Source: CAD feature listing. Evaluate the final solid. Frame: model axes, mm. Face numbers are marked on the shaded views. A direction names the side the tool comes from. Give positions to 0.01 mm unless a question says otherwise; leave off trailing zeros. Write each loop counter-clockwise with the first axis right and the second up, starting at its lowest first coordinate (ties: lowest second). Pieces come first, ordered by that corner, then holes. Notation, with made-up numbers: (48, -26.5) -> (66, -26.5) arc R21 ccw to (66, 11.5) -> close; hole circle Ø1 at (30, -1.75). An arc over 180 degrees is marked (long way). Write item = value, one per line.
Autodesk Inventor part; units mm, degrees
ref_plane "YZ Plane" through (0, 0, 0) normal (1, 0, 0) x (0, 1, 0)
ref_plane "XZ Plane" through (0, 0, 0) normal (0, 1, 0) x (-1, 0, 0)
ref_plane "XY Plane" through (0, 0, 0) normal (0, 0, 1) x (1, 0, 0)
sketch "Sketch1" plane through (0, 0, 0) normal (0, 1, 0) x (-1, 0, 0)
  line L0 (0, 0) -> (850, 0)
  line L1 (850, 0) -> (850, 850)
  line L2 (850, 850) -> (0, 850)
  line L3 (0, 850) -> (0, 0)
  dimension "d0" = 850
  dimension "d1" = 850
extrude "Extrusion1" add sketch "Sketch1" along normal blind 950
sketch "Sketch2" plane through (0, 950, 0) normal (0, 1, 0) x (1, 0, 0)
  line L0 (0, 0) -> (-850, 0)
  line L1 (-850, 0) -> (-850, -850)
  line L2 (-850, -850) -> (0, -850)
  line L3 (0, -850) -> (0, 0)
  line L4 (-810, -40) -> (-40, -40)
  line L5 (-40, -40) -> (-40, -810)
  line L6 (-40, -810) -> (-810, -810)
  line L7 (-810, -810) -> (-810, -40)
  dimension "d4" = 40
extrude "Extrusion2" cut sketch "Sketch2" against normal blind 1000 contours L4 L5 L6 L7
sketch "Sketch3" plane through (-850, 0, 850) normal (0, 0, 1) x (1, 0, 0)
  line L0 (0, 0) -> (850, 0)
  line L1 (850, 0) -> (850, 950)
  line L2 (0, 950) -> (850, 950)
  line L3 (0, 0) -> (0, 950)
  line L4 (0, 2.54) -> (850, 2.54)
  line L5 (850, 2.54) -> (850, 947.46)
  line L6 (850, 947.46) -> (0, 947.46)
  line L7 (0, 947.46) -> (0, 2.54)
  dimension "d7" = 2.54
  dimension "d8" = 2.54
extrude "Extrusion3" cut sketch "Sketch3" against normal blind 37.5 contours L3 L6 L1 L4
sketch "Sketch4" plane through (0, 0, 0) normal (0, 0, -1) x (-1, 0, 0)
  line L0 (0, 0) -> (850, 0)
  line L1 (850, 0) -> (850, 950)
  line L2 (0, 950) -> (850, 950)
  line L3 (0, 0) -> (0, 950)
  line L4 (0, 2.54) -> (850, 2.54)
  line L5 (850, 2.54) -> (850, 947.46)
  line L6 (850, 947.46) -> (0, 947.46)
  line L7 (0, 947.46) -> (0, 2.54)
  dimension "d11" = 2.54
  dimension "d12" = 2.54
extrude "Extrusion4" cut sketch "Sketch4" against normal blind 37.5 contours L3 L6 L1 L4
sketch "Sketch5" plane through (0, 0, 37.5) normal (0, 0, -1) x (-1, 0, 0)
  line L0 (850, 2.54) -> (0, 2.54)
  line L1 (0, 947.46) -> (37.5, 947.46)
  line L2 (37.5, 947.46) -> (37.5, 2.54)
  line L3 (37.5, 2.54) -> (0, 2.54)
  line L4 (0, 2.54) -> (0, 947.46)
  line L5 (850, 947.46) -> (812.5, 947.46)
  line L6 (812.5, 947.46) -> (812.5, 2.54)
  line L7 (812.5, 2.54) -> (850, 2.54)
  line L8 (850, 2.54) -> (850, 947.46)
  point P0 (0, 0)
  dimension "d15" = 37.5
  dimension "d16" = 37.5
extrude "Extrusion5" cut sketch "Sketch5" against normal blind 1000
sketch "Sketch6" plane through (0, 950, 0) normal (0, 1, 0) x (1, 0, 0)
  line L0 (0, 0) -> (-850, 0)
  line L1 (-850, 0) -> (-850, -850)
  circle A0 centre (-835, -15) radius 5.0825
  point P0 (-165, -15)
  point P1 (-835, -685)
  point P2 (-165, -685)
  dimension "d19" = 15
  dimension "d20" = 15
  dimension "d23" = 670
  dimension "d26" = 670
hole "Hole1" at (-835, 950, 685) at (-835, 950, 15) at (-165, 950, 15) at (-165, 950, 685) direction (0, -1, 0) diameter 6.35 end through all
sketch "Sketch7" plane through (0, 0, 37.5) normal (0, 0, -1) x (-1, 0, 0)
  line L0 (37.5, 947.46) -> (37.5, 2.54)
  line L1 (257.5, 604.8881) -> (437.5, 604.8881)
  line L2 (437.5, 604.8881) -> (437.5, 784.8881)
  line L3 (437.5, 784.8881) -> (257.5, 784.8881)
  line L4 (257.5, 784.8881) -> (257.5, 604.8881)
  point P0 (0, 0)
  dimension "d36" = 220
  dimension "d37" = 180
  dimension "d38" = 180
extrude "Extrusion6" cut sketch "Sketch7" against normal blind 10
properties part number "housing" material "Aluminum 6061"
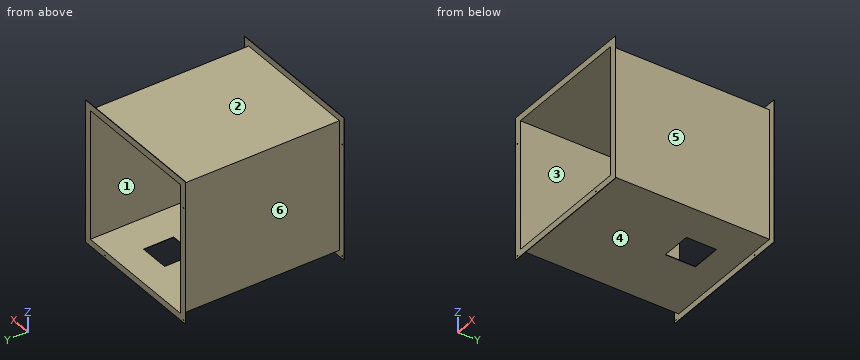
1) Contact query for flat-ended pins moving along their axis: pin 1 (12 mm diameter, centred on x = -316, y = 453.5, fed in from +Z); pin 2 (2 mm diameter, centred on y = 671, z = 39, fed in from +X); pin 3 (1.5 mm diameter, centred on y = 640, z = 754.5, fed in from -X); pin 4 (10 mm diameter, centred on x = -835, z = 685, fed in from -Y). Output: stop coordinate, or through.
Computed:
pin_1 = 812.5
pin_2 = -37.5
pin_3 = -812.5
pin_4 = 0
2) Cut plane A-A (z = 255). Return the cut outline in (x, y).
Computed:
outline = (-850, 0) -> (-810, 0) -> (-810, 950) -> (-850, 950) -> (-850, 947.46) -> (-812.5, 947.46) -> (-812.5, 2.54) -> (-850, 2.54) -> close; (-40, 0) -> (0, 0) -> (0, 2.54) -> (-37.5, 2.54) -> (-37.5, 947.46) -> (0, 947.46) -> (0, 950) -> (-40, 950) -> close
3) Material intervals for L1, parallel to Z at x = -835, y = 1 (3 decimals); L2, parallel to X at y = 1, z = 15 (3 decimals); L3, parallel to X at y = 346, z = 331, sorted ascending.
Computed:
L1 = 0 to 11.825, 18.175 to 681.825, 688.175 to 850
L2 = -850 to -838.175, -831.825 to -168.175, -161.825 to 0
L3 = -812.5 to -810, -40 to -37.5
4) Cut plane B-B (x = -121). Return the cut outline in (y, z).
Computed:
outline = (0, 0) -> (2.54, 0) -> (2.54, 37.5) -> (947.46, 37.5) -> (947.46, 0) -> (950, 0) -> (950, 40) -> (0, 40) -> close; (0, 810) -> (950, 810) -> (950, 850) -> (947.46, 850) -> (947.46, 812.5) -> (2.54, 812.5) -> (2.54, 850) -> (0, 850) -> close
5) Draft query along X for the marked faces 3, 4, 5 and 6. Return one class per face: pulls with the +X half, pulls with the -X half, needs draft (parallel to the pull), parting line crosses it, or undercut.
Computed:
face_3 = undercut
face_4 = needs draft
face_5 = pulls with the +X half
face_6 = pulls with the -X half
6) Cut plane C-C (y = 109). Return the cut outline in (x, z), then the cut area to 4 significant figures.
Computed:
outline = (-812.5, 37.5) -> (-37.5, 37.5) -> (-37.5, 812.5) -> (-812.5, 812.5) -> close; hole (-810, 40) -> (-40, 40) -> (-40, 810) -> (-810, 810) -> close
area = 7,725 mm²
7) Access query for the marked faces 1 and 2. Directions: +Z, -Z, +X, -X, +Y, -Y. A direction counts if a zero-diameter tool reaches every point of the face in a straight line with its end or side. Return the directions, or none.
Computed:
face_1 = +Y, -Y
face_2 = +Z, +X, -X
